```python
from build123d import *

# Parameters (mm, degrees)
F0_R     = 5.55625
F1_DEPTH = 0.79375
F2_R     = 3.175
F3_DEPTH = 1.5885
F4_R     = 0.508


with BuildPart() as f1:
    # F0 (on Top) → F1 (new body, symmetric)
    with BuildSketch(Plane.XY):
        Circle(F0_R)
    extrude(amount=F1_DEPTH, both=True)

    # F2 (on face) → F3 (cut, through all)
    with BuildSketch(Plane.XY.offset(0.79375)):
        Circle(F2_R)
    extrude(amount=-F3_DEPTH, mode=Mode.SUBTRACT)

    # F4
    f4_edges = [f1.edges().sort_by_distance(p)[0] for p in [
        (-5.55625, 0, 0.79375),
        (-5.55625, 0, -0.79375),
    ]]
    fillet(f4_edges, radius=F4_R)


solid = f1.part
```
Geometry check sheet. Reference: the model listing, model coordinates, mm. Coordinates: 2 decimals unless noted, no trailing zeros. Loops run counter-clockwise (first coordinate to the right, second up) from the corner with the lowest first, then second, coordinate; pieces in that order, holes last. Notation, with made-up numbers: (34, 51.25) -> (86, 51.25) arc R16 ccw to (86, 72.25) -> close; hole circle Ø8 at (47.5, -37). An arc over 180 degrees is marked (long way). Put each result on its own line as item: value.
1) Cross-section at A-A on y = 0. Record the boundary of the cut face in (x, z) (3 decimals), plus the area to 3 significant figures.
Result set:
outline: (-5.556, -0.286) arc R0.508 ccw to (-5.048, -0.794) -> (-3.175, -0.794) -> (-3.175, 0.794) -> (-5.048, 0.794) arc R0.508 ccw to (-5.556, 0.286) -> close; (3.175, -0.794) -> (5.048, -0.794) arc R0.508 ccw to (5.556, -0.286) -> (5.556, 0.286) arc R0.508 ccw to (5.048, 0.794) -> (3.175, 0.794) -> close
area: 7.34 mm^2
2) Gauge pin test, flat end, axial feed: pin 1 Ø5 at (x, y) = (-1.5, 0.5) entering from -Z. Record the tip position at first contact, or that the pin passes through.
Result set:
pin 1: stops at z = -0.79
3) Release check for a two-part mould opening along Y. For faces 1 (the flat face through (3.3, -1.1, 0.794)), 2 (the cylindrical face through (-0.69, -3.1, 0.01)), 3 (the cylindrical face through (5.3, 1.67, 0)) record: released by +Y, released by -Y, zero draft, split by the parting line, or undercut.
Result set:
face 1: zero draft
face 2: undercut
face 3: split by the parting line
4) Thickness scan on line 1 (Y direction, x = 0, z = 0.25) (3 decimals); line 2 (Y direction, x = 1.5, z = 0.5); line 3 (X direction, y = 0.25, z = -0.5). Record the ranges inside material, lowest first.
Result set:
line 1: y = -5.556 to -3.175, 3.175 to 5.556
line 2: y = -5.3 to -2.8, 2.8 to 5.3
line 3: x = -5.5 to -3.17, 3.17 to 5.5
5) Cross-section at D-D on z = 0.45. Record the boundary of the cut face in (x, y) (3 decimals), plus the area to 3 significant figures.
Result set:
outline: circle Ø11.058 at (0, 0); hole circle Ø6.35 at (0, 0)
area: 64.4 mm^2
